Here's how the part is built. I have some questions about the finished solid (model axes, mm). A direction names the side the tool comes from. Coordinates: 2 decimals unless noted, no trailing zeros. Loops run counter-clockwise (first coordinate to the right, second up) from the corner with the lowest first, then second, coordinate; pieces in that order, holes last. Notation, with made-up numbers: (-26, 3.25) -> (1, 3.25) arc R14 cw to (1, 17.25) -> close; hole circle Ø3 at (78.5, 88.25). An arc over 180 degrees is marked (long way). Answer as a JSON object with one key per item and string values. Group by question number.
Q1. I'm going to push flat-ended pins straight in: pin 1 (1.6 mm diameter, centred on y = -20, z = 1.5, fed in from -X); pin 2 (1.5 mm diameter, centred on x = 29.5, z = 1.5, fed in from -Y); pin 3 (1 mm diameter, centred on y = -20.5, z = 2, fed in from +X). Where does each tip first touch, or does it pass through?
Q2. I want a section at A-A on x = 0. Write out the boundary of the cut face in (y, z), then the cut area to 3 significant figures.
Q3. I need wall thicknesses on line 1 (X direction, y = -29.25, z = 2.6); line 2 (X direction, y = -17.75, z = 0.45); line 3 (Y direction, x = 0, z = 0.7). Which ranges of each line are inside material? Lowest first, please.
Q4. I want a section at D-D on z = 0.8. Count the separate pieces of the cut face and the enclosed holes in it, then the cut area to 3 significant figures.
Q5. On a 3-axis mill with a long thin cutter (end or side, diameter ignored), from which of +Z, -Z, +X, -X, +Y, -Y can I reach the whole of each face in a straight line? I mean faces 1 (the flat face through (29, -24.604, 1)), 2 (the flat face through (-14.029, -19.634, 1.479)), 3 (the flat face through (28, -37, 1)), 4 (the flat face through (-30, -33.604, 1)), 5 (the cylindrical face through (23.43, -35.08, 1.52)). Say none if no direction works.
Q6. I want a section at C-C on x = -13.5. Write out the boundary of the cut face in (y, z), then the cut area to 3 significant figures.
Q7. I want a section at B-B on y = -20. Write out the boundary of the cut face in (x, z).
Q8. Thinking about a two-plate mould opening in Y: for faces 6 (the cylindrical face through (6.02, -28.9, 1.52)), 7 (the flat face through (26, -20, 2)), 8 (the flat face through (-2, -33, 3)), 9 (the flat face through (0, -41.207, 1)), which applies, released by +Y, released by -Y, zero draft, split by the parting line, or undercut?
Autodesk Inventor part; units mm, degrees
ref_plane "YZ Plane" through (0, 0, 0) normal (1, 0, 0) x (0, 1, 0)
ref_plane "XZ Plane" through (0, 0, 0) normal (0, 1, 0) x (-1, 0, 0)
ref_plane "XY Plane" through (0, 0, 0) normal (0, 0, 1) x (1, 0, 0)
sketch "スケッチ1" plane through (0, 0, 0) normal (0, 0, 1) x (1, 0, 0)
  line L0 (0, 0) -> (0, 4) construction
  line L1 (0, 0) -> (8.6476, -12.2564)
  line L2 (8.6476, -12.2564) -> (-0.2755, 4.5179)
  circle A0 centre (3.0119, -1.6621) radius 4
  line L3 (-57.3278, -140) -> (69.8706, -140)
  line L4 (3.0119, -1.6621) -> (117.7837, 59.3906)
  circle A1 centre (0, 0) radius 23.1
  circle A2 centre (0, -29.1039) radius 6.0039
  line L5 (0, 0) -> (0, -29.1039) construction
  circle A3 centre (0, -29.1039) radius 16.55
  circle A4 centre (0, -7.5039) radius 5.05
  circle A5 centre (0, 4) radius 3
  circle A6 centre (0, -7.5039) radius 20.05
  circle A7 centre (-14, 10.2376) radius 2.55
  circle A8 centre (14, 10.2376) radius 2.55
  circle A9 centre (14, -25.2454) radius 2.55
  circle A10 centre (-14, -25.2454) radius 2.55
  circle A11 centre (-14, 10.2376) radius 14
  circle A12 centre (14, 10.2376) radius 14
  circle A13 centre (14, -25.2454) radius 14
  circle A14 centre (-14, -25.2454) radius 14
  line L6 (-14, 10.2376) -> (-14, -25.2454) construction
  line L7 (-14, -25.2454) -> (14, -25.2454) construction
  circle A15 centre (0, 0) radius 9
  line L8 (-0.2755, 4.5179) -> (3.4816, -2.5449) construction
  line L9 (-2.9462, 3.0973) -> (0.8109, -3.9656)
  line L10 (6.1522, -1.1243) -> (2.3951, 5.9386)
  arc A16 (2.3951, 5.9386) -> (-2.9462, 3.0973) centre (-0.2755, 4.5179) ccw
  arc A17 (0.8109, -3.9656) -> (6.1522, -1.1243) centre (3.4816, -2.5449) ccw
  line L11 (-5, 2.8868) -> (5, 2.8868) construction
  line L12 (5, 2.8868) -> (0, -5.7735) construction
  line L13 (0, -5.7735) -> (-5, 2.8868) construction
  circle A18 centre (-5, 2.8868) radius 1.5
  circle A19 centre (5, 2.8868) radius 1.5
  circle A20 centre (0, -5.7735) radius 1.5
  line L14 (-28, 22.5965) -> (-28, -43.3295)
  line L15 (28, 22.9271) -> (28, -43.0008)
  line L16 (-28, 26.1991) -> (28, 26.1991)
  circle A21 centre (0, 0) radius 25.1
  line L17 (-28, -18.848) -> (28, -18.848)
  circle A22 centre (0, -29.1039) radius 8.0039
  circle A23 centre (-25, 23.1991) radius 3
  circle A24 centre (25, 23.1991) radius 3
  circle A25 centre (25, -38.2069) radius 3
  circle A26 centre (-25, -38.2069) radius 3
  circle A27 centre (-25, -15.848) radius 3
  circle A28 centre (25, -15.848) radius 3
  circle A29 centre (-25, -15.848) radius 4.5
  circle A30 centre (25, -15.848) radius 4.5
  circle A31 centre (0, -7.5039) radius 4.5
  circle A32 centre (0, -29.1039) radius 17.55
  circle A33 centre (0, -7.5039) radius 6.05
  point P0 (1.603, 0.9865)
  dimension "d0" = 4
  dimension "d1" = 15
  dimension "d2" = 18.4133
  dimension "d3" = 19
  dimension "d4" = 8
  dimension "d5" = 12
  dimension "d6" = 140
  dimension "d7" = 130
  dimension "d8" = 46.2
  dimension "d9" = 29.1039
  dimension "d10" = 33.1
  dimension "d11" = 10.1
  dimension "d12" = 6
  dimension "d13" = 40.1
  dimension "d14" = 28
  dimension "d15" = 28
  dimension "d16" = 28
  dimension "d17" = 28
  dimension "d18" = 18
  dimension "d19" = 8
  dimension "d20" = 6.05
  dimension "d21" = 3
  dimension "d22" = 3
  dimension "d23" = 3
  dimension "d24" = 10
  dimension "d25" = 2
  dimension "d26" = 2
  dimension "d27" = 6
  dimension "d28" = 6
  dimension "d29" = 6
  dimension "d30" = 6
  dimension "d31" = 6
  dimension "d32" = 6
  dimension "d33" = 9
  dimension "d34" = 9
  dimension "d35" = 9
  dimension "d36" = 5.1
  dimension "d37" = 1
  dimension "d38" = 1
  dimension "d39" = 56
  dimension "d40" = 28
sketch "スケッチ2" plane through (0, 0, 0) normal (0, 0, 1) x (1, 0, 0)
  circle A0 centre (-25, -15.848) radius 3
  circle A1 centre (-25, -38.2069) radius 3
  circle A2 centre (25, -38.2069) radius 3
  circle A3 centre (25, -15.848) radius 3
  circle A4 centre (0, -29.1039) radius 6.0039 construction
  circle A5 centre (0, 0) radius 25.1 construction
  circle A6 centre (0, -29.1039) radius 4.025
  line L0 (25, -41.2069) -> (-25, -41.2069)
  circle A7 centre (-25, -15.848) radius 1.5
  circle A8 centre (25, -15.848) radius 1.5
  circle A9 centre (25, -38.2069) radius 1.5
  circle A10 centre (-25, -38.2069) radius 1.5
  circle A11 centre (0, -29.1039) radius 6.025
  line L1 (23.3216, -13.3615) -> (4.9938, -25.733)
  line L2 (-4.9938, -25.733) -> (-23.3216, -13.3615)
  line L3 (-28, -15.848) -> (-28, -38.2069)
  line L4 (28, -15.848) -> (28, -38.2069)
  line L5 (-28, -24.6039) -> (-31, -24.6039)
  line L6 (-31, -24.6039) -> (-31, -33.6039)
  line L7 (-31, -33.6039) -> (-28, -33.6039)
  line L8 (28, -24.6039) -> (31, -24.6039)
  line L9 (31, -24.6039) -> (31, -33.6039)
  line L10 (31, -33.6039) -> (28, -33.6039)
  circle A12 centre (-28, -34.6539) radius 1.05
  circle A13 centre (-28, -23.5539) radius 1.05
  circle A14 centre (28, -23.5539) radius 1.05
  circle A15 centre (28, -34.6539) radius 1.05
  point P0 (-28, -22.5039)
  point P1 (-28, -35.7039)
  point P2 (28, -35.7039)
  point P3 (28, -22.5039)
  dimension "d41" = 8.05
  dimension "d52" = 3
  dimension "d53" = 3
  dimension "d54" = 3
  dimension "d55" = 3
  dimension "d57" = 2
  dimension "d61" = 3
  dimension "d62" = 9
  dimension "d63" = 3
  dimension "d64" = 9
  dimension "d65" = 2.1
  dimension "d66" = 2.1
  dimension "d67" = 2.1
  dimension "d68" = 2.1
  dimension "d69" = 4.5
extrude "押し出し2" add sketch "スケッチ2" along normal blind 3 contours A0 | A0 L2 A11 L1 A3 L4 A14 A15 A2 L0 A1 L3 A12 A13 | A11 | L3 L7 L6 L5 | A3 | A1 | L8 L9 L10 L4 | A2
sketch "スケッチ3" plane through (0, 0, 3) normal (0, 0, 1) x (1, 0, 0)
  line L0 (-28, -15.848) -> (-28, -22.5039)
  arc A0 (-28, -24.6039) -> (-28, -22.5039) centre (-28, -23.5539) ccw
  line L1 (-28, -24.6039) -> (-31, -24.6039)
  line L2 (-31, -24.6039) -> (-31, -33.6039)
  line L3 (-31, -33.6039) -> (-28, -33.6039)
  arc A1 (-28, -35.7039) -> (-28, -33.6039) centre (-28, -34.6539) ccw
  line L4 (-28, -35.7039) -> (-28, -38.2069)
  arc A2 (-28, -38.2069) -> (-25, -41.2069) centre (-25, -38.2069) ccw
  line L5 (-25, -41.2069) -> (25, -41.2069)
  arc A3 (25, -41.2069) -> (28, -38.2069) centre (25, -38.2069) ccw
  line L6 (28, -38.2069) -> (28, -35.7039)
  arc A4 (28, -33.6039) -> (28, -35.7039) centre (28, -34.6539) ccw
  line L7 (28, -33.6039) -> (31, -33.6039)
  line L8 (31, -33.6039) -> (31, -24.6039)
  line L9 (31, -24.6039) -> (28, -24.6039)
  arc A5 (28, -22.5039) -> (28, -24.6039) centre (28, -23.5539) ccw
  line L10 (28, -22.5039) -> (28, -15.848)
  arc A6 (28, -15.848) -> (23.3216, -13.3615) centre (25, -15.848) ccw
  line L11 (23.3216, -13.3615) -> (4.9938, -25.733)
  arc A7 (4.9938, -25.733) -> (-4.9938, -25.733) centre (0, -29.1039) ccw
  line L12 (-4.9938, -25.733) -> (-23.3216, -13.3615)
  arc A8 (-23.3216, -13.3615) -> (-28, -15.848) centre (-25, -15.848) ccw
  circle A9 centre (25, -38.2069) radius 1.5
  circle A10 centre (-25, -38.2069) radius 1.5
  circle A11 centre (25, -15.848) radius 1.5
  circle A12 centre (0, -29.1039) radius 4.025
  circle A13 centre (-25, -15.848) radius 1.5
  line L13 (-24.4405, -15.0192) -> (-4.0141, -28.8074)
  arc A14 (4.0141, -28.8074) -> (-4.0141, -28.8074) centre (0, -29.1039) ccw
  line L14 (4.0141, -28.8074) -> (24.4405, -15.0192)
  arc A15 (26, -15.848) -> (24.4405, -15.0192) centre (25, -15.848) ccw
  line L15 (26, -15.848) -> (26, -21.2512)
  arc A16 (26, -21.2512) -> (28, -26.6039) centre (28, -23.5539) ccw
  line L16 (28, -26.6039) -> (29, -26.6039)
  line L17 (29, -26.6039) -> (29, -31.6039)
  line L18 (29, -31.6039) -> (28, -31.6039)
  arc A17 (28, -31.6039) -> (26, -36.9566) centre (28, -34.6539) ccw
  line L19 (26, -36.9566) -> (26, -38.2069)
  arc A18 (25, -39.2069) -> (26, -38.2069) centre (25, -38.2069) ccw
  line L20 (25, -39.2069) -> (-25, -39.2069)
  arc A19 (-26, -38.2069) -> (-25, -39.2069) centre (-25, -38.2069) ccw
  line L21 (-26, -38.2069) -> (-26, -36.9566)
  arc A20 (-26, -36.9566) -> (-28, -31.6039) centre (-28, -34.6539) ccw
  line L22 (-28, -31.6039) -> (-29, -31.6039)
  line L23 (-29, -31.6039) -> (-29, -26.6039)
  line L24 (-29, -26.6039) -> (-28, -26.6039)
  arc A21 (-28, -26.6039) -> (-26, -21.2512) centre (-28, -23.5539) ccw
  line L25 (-26, -21.2512) -> (-26, -15.848)
  arc A22 (-24.4405, -15.0192) -> (-26, -15.848) centre (-25, -15.848) ccw
  circle A23 centre (0, -29.1039) radius 6.025
  circle A24 centre (25, -15.848) radius 3.5
  circle A25 centre (25, -38.2069) radius 3.5
  circle A26 centre (-25, -38.2069) radius 3.5
  circle A27 centre (-25, -15.848) radius 3.5
  line L26 (-25, -38.2069) -> (0, -29.1039) construction
  line L27 (-24.6579, -39.1465) -> (0.3421, -30.0435)
  line L28 (-0.3421, -28.1643) -> (-25.3421, -37.2672)
  arc A28 (-25.3421, -37.2672) -> (-24.6579, -39.1465) centre (-25, -38.2069) ccw
  arc A29 (0.3421, -30.0435) -> (-0.3421, -28.1643) centre (0, -29.1039) ccw
  line L29 (0, -29.1039) -> (25, -38.2069) construction
  line L30 (-0.3421, -30.0435) -> (24.6579, -39.1465)
  line L31 (25.3421, -37.2672) -> (0.3421, -28.1643)
  arc A30 (0.3421, -28.1643) -> (-0.3421, -30.0435) centre (0, -29.1039) ccw
  arc A31 (24.6579, -39.1465) -> (25.3421, -37.2672) centre (25, -38.2069) ccw
  line L32 (-28, -22.5039) -> (-28, -35.7039)
  line L33 (28, -38.2069) -> (28, -35.7039)
  line L34 (28, -22.5039) -> (28, -35.7039)
  point P0 (0, 0)
  point P1 (-12.5, -33.6554)
  point P2 (12.5, -33.6554)
  point P3 (28, -26.6039)
  point P4 (26, -19.2021)
  point P5 (21.6605, -16.8957)
  point P6 (5.8296, -27.5818)
  point P7 (5.925, -30.1971)
  point P8 (22.1905, -36.1196)
  point P9 (24.9505, -34.7072)
  point P10 (21.5062, -37.9989)
  point P11 (5.2407, -32.0764)
  point P12 (-5.2407, -32.0764)
  point P13 (-21.5062, -37.9989)
  point P14 (-21.6459, -39.2069)
  point P15 (21.6459, -39.2069)
  point P16 (-28, -31.6039)
  point P17 (-24.9505, -34.7072)
  point P18 (-22.1905, -36.1196)
  point P19 (-5.925, -30.1971)
  point P20 (-5.8296, -27.5818)
  point P21 (-21.6605, -16.8957)
  point P22 (-26, -19.2021)
  dimension "d72" = 2
  dimension "d73" = 2
  dimension "d74" = 2
  dimension "d75" = 2
  dimension "d76" = 2
  dimension "d77" = 2
  dimension "d78" = 2
  dimension "d79" = 2
extrude "押し出し3" cut sketch "スケッチ3" against normal blind 10 contours A27 L13 A23 L28 A26 A20 L32 A21 L25 | L14 A24 L15 A16 L34 A17 A25 L31 A23 | A23 L30 A25 L20 A26 L27
equation "\"d14\" = d15"
equation "\"d16\" = d15"
equation "\"d17\" = d14"
equation "\"d40\" = 0.5 * d39"
properties part number "横回転フレーム改３" material "アルミニウム 2014-T4"
Result set:
{
 "1": {"pin 1": "stops at x = -28", "pin 2": "stops at y = -33.6", "pin 3": "stops at x = 28"},
 "2": {"outline": "(-41.21, 0) -> (-39.21, 0) -> (-39.21, 3) -> (-41.21, 3) -> close; (-35.13, 0) -> (-33.13, 0) -> (-33.13, 3) -> (-35.13, 3) -> close; (-25.08, 0) -> (-23.08, 0) -> (-23.08, 3) -> (-25.08, 3) -> close", "area": "18.0 mm²"},
 "3": {"line 1": "x = -31 to -28, -6.02 to -4.02, 4.02 to 6.02, 28 to 31", "line 2": "x = -28 to -22.06, -20.39 to -16.82, 16.82 to 20.39, 22.06 to 28", "line 3": "y = -41.21 to -39.21, -35.13 to -33.13, -25.08 to -23.08"},
 "4": {"separate pieces": "1", "enclosed holes": "8", "area": "510 mm²"},
 "5": {"face 1": "+Z, -Z, +X, +Y", "face 2": "+Z, -Z, +Y", "face 3": "+Z, -Z, +X, -Y", "face 4": "+Z, -Z, -X, -Y", "face 5": "+Z, -Z"},
 "6": {"outline": "(-41.21, 0) -> (-39.21, 0) -> (-39.21, 3) -> (-41.21, 3) -> close; (-35.08, 0) -> (-32.96, 0) -> (-32.96, 3) -> (-35.08, 3) -> close; (-22.4, 0) -> (-19.99, 0) -> (-19.99, 3) -> (-22.4, 3) -> close", "area": "19.6 mm²"},
 "7": {"outline": "(-28, 0) -> (-26, 0) -> (-26, 3) -> (-28, 3) -> close; (-17.06, 0) -> (-13.49, 0) -> (-13.49, 3) -> (-17.06, 3) -> close; (13.49, 0) -> (17.06, 0) -> (17.06, 3) -> (13.49, 3) -> close; (26, 0) -> (28, 0) -> (28, 3) -> (26, 3) -> close"},
 "8": {"face 6": "undercut", "face 7": "undercut", "face 8": "zero draft", "face 9": "released by -Y"}
}
